Part model, mm, in its own coordinate system. A direction names the side the tool comes from. Coordinates: 2 decimals unless noted, no trailing zeros. Loops run counter-clockwise (first coordinate to the right, second up) from the corner with the lowest first, then second, coordinate; pieces in that order, holes last. Notation, with made-up numbers: M 62.25,39.25 L 75.25,39.25 A25 cw 75.25,62.25 Z; hole C 35.25,14 d9. An arc over 180 degrees is marked long. Answer as a JSON object with one key per item and string values. Group by question number.
1. Saw through at C-C on y = -2.5. Write the cut outline in (x, z), then the cut area to 3 significant figures.
2. Saw through at D-D on x = 0. Write the cut outline in (y, z).
3. Saw through at B-B on z = 0.85. Count the separate pieces of the cut face and the enclosed holes in it, then the cut area to 3 significant figures.
4. Drill centre lines: L1, parallel to X at y = -0.25, z = 2.45; L2, parallel to Y at x = 0, z = 2.6; L3, parallel to Y at x = 5, z = 3.55. Where is each one in solid material? Low to high.
5. 3-axis set-ups, long thin cutter, end or side, ignore diameter. For faces 5 (the face through (16.96, 6.08, 3.04)), 6 (the face through (-16.95, -5.32, 3.04)), 7 (the face through (0, 11, 3)), 8 (the face through (4.2, -2, 3)): which of +Z, -Z, +X, -X, +Y, -Y reach the whole face in a straight line?
6. Mould opens along X. For faces 1 (the face through (0, 2, 0)), 2 (the face through (17.2, 8, 3)), 3 (the face through (5, -5, 3)), 4 (the face through (-17.2, -6.5, 3)) say: released by +X, released by -X, zero draft, split by the parting line, or undercut.
7. Drop flat-ended pins along their axis: pin 1 Ø3.5 at (y, z) = (-1, 3) entering from +X; pin 2 Ø1.8 at (x, y) = (0, -2) entering from -Z; pin 3 Ø2 at (y, z) = (-1.5, 3.5) entering from -X; pin 4 Ø3 at (y, z) = (4.5, 3.5) entering from +X. Give the stop position or say it passes through.
8. Saw through at A-A on x = 4.95. Write the cut outline in (y, z).
from build123d import *

# Parameters (mm, degrees)
F0_R     = 1.5
F1_DEPTH = 6
F2_R     = 1
F3_R     = 1


with BuildPart() as f1:
    # F0 (on Top) → F1 (new body)
    with BuildSketch(Plane.XY):
        with BuildLine():
            Line((17.2, 11), (-17.2, 11))
            Line((-17.2, 11), (-17.2, 5.0637826232))
            ThreePointArc((-17.2, 5.0637826232), (-16.4207968358, 5.7493204245), (-15.7027170703, 5))
            Line((-15.7027170703, 5), (-15.7027170703, -4.25))
            ThreePointArc((-15.7027170703, -4.25), (-16.4207968358, -4.9993204245), (-17.2, -4.3137826232))
            Line((-17.2, -4.3137826232), (-17.2, -8))
            Line((-17.2, -8), (17.2, -8))
            Line((17.2, -8), (17.2, -4.25))
            ThreePointArc((17.2, -4.25), (16.45, -5), (15.7, -4.25))
            Line((15.7, -4.25), (15.7, 5))
            ThreePointArc((15.7, 5), (16.45, 5.75), (17.2, 5))
            Line((17.2, 5), (17.2, 11))
        make_face()
        with BuildLine():
            Line((-5.7027170703, -4.25), (-5.7027170703, 0.25))
            ThreePointArc((-5.7027170703, 0.25), (-4.9527170703, 1), (-4.2027170703, 0.25))
            Line((-4.2027170703, 0.25), (-4.2027170703, -4.25))
            ThreePointArc((-4.2027170703, -4.25), (-4.9527170703, -5), (-5.7027170703, -4.25))
        make_face(mode=Mode.SUBTRACT)
        with Locations((0, -2)):
            Circle(F0_R, mode=Mode.SUBTRACT)
        with BuildLine():
            Line((4.2, -4.25), (4.2, 0.25))
            ThreePointArc((4.2, 0.25), (4.95, 1), (5.7, 0.25))
            Line((5.7, 0.25), (5.7, -4.25))
            ThreePointArc((5.7, -4.25), (4.95, -5), (4.2, -4.25))
        make_face(mode=Mode.SUBTRACT)
    extrude(amount=F1_DEPTH)

    # F2
    f2_edges = [f1.edges().sort_by_distance(p)[0] for p in [
        (17.2, 11, 3),
        (17.2, -8, 3),
        (-17.2, -8, 3),
        (-17.2, 11, 3),
    ]]
    fillet(f2_edges, radius=F2_R)

    # F3
    f3_edges = [f1.edges().sort_by_distance(p)[0] for p in [
        (17.2, 5, 3),
        (17.2, -4.25, 3),
        (-17.2, 5.063783, 3),
        (-17.2, -4.313783, 3),
    ]]
    fillet(f3_edges, radius=F3_R)


solid = f1.part
Outcome:
{
 "1": {"outline": "M -15.7,0 L -5.7,0 L -5.7,6 L -15.7,6 Z; M -4.2,0 L -1.41,0 L -1.41,6 L -4.2,6 Z; M 1.41,0 L 4.2,0 L 4.2,6 L 1.41,6 Z; M 5.7,0 L 15.7,0 L 15.7,6 L 5.7,6 Z", "area": "153 mm²"},
 "2": {"outline": "M -8,0 L -3.5,0 L -3.5,6 L -8,6 Z; M -0.5,0 L 11,0 L 11,6 L -0.5,6 Z"},
 "3": {"separate pieces": "1", "enclosed holes": "3", "area": "596 mm²"},
 "4": {"L1": "x = -15.7 to -5.7, -4.2 to 4.2, 5.7 to 15.7", "L2": "y = -8 to -3.5, -0.5 to 11", "L3": "y = -8 to -5, 1 to 11"},
 "5": {"face 5": "+Z, -Z, +X", "face 6": "+Z, -Z, -X", "face 7": "+Z, -Z, +X, -X, +Y", "face 8": "+Z, -Z"},
 "6": {"face 1": "zero draft", "face 2": "released by +X", "face 3": "undercut", "face 4": "released by -X"},
 "7": {"pin 1": "stops at x = 15.7", "pin 2": "passes through", "pin 3": "stops at x = -15.7", "pin 4": "stops at x = 16.88"},
 "8": {"outline": "M -8,0 L -5,0 L -5,6 L -8,6 Z; M 1,0 L 11,0 L 11,6 L 1,6 Z"}
}
